```python
from build123d import *

# Parameters (mm, degrees)
SKETCH1_W           = 30
SKETCH1_H           = 20
SKETCH1_H_2         = 2.5
SKETCH1_W_2         = 14
SKETCH1_W_3         = 13.5
SKETCH1_H_3         = 5
SKETCH1_W_4         = 2.5
BOSS_EXTRUDE1_DEPTH = 5
SKETCH1_3_W         = 13.5
SKETCH1_3_H         = 2.5
SKETCH1_3_W_2       = 14
SKETCH1_3_W_3       = 30
SKETCH1_3_W_4       = 2.5
BOSS_EXTRUDE2_DEPTH = 8
SKETCH3_R           = 1.5
CUT_EXTRUDE2_DEPTH  = 2.5
CUT_EXTRUDE3_DEPTH  = 2.5
CUT_EXTRUDE1_DEPTH  = 43.720018727
CUT_EXTRUDE4_DEPTH  = 2.5


with BuildPart() as part:
    # Sketch1 → Boss-Extrude1 (new body)
    with BuildSketch(Plane(origin=(0, 0, 0), x_dir=(1, 0, 0), z_dir=(0, 1, 0))):
        with Locations((-15, -10)):
            Rectangle(SKETCH1_W, SKETCH1_H)
        with Locations((-15, -21.25)):
            Rectangle(SKETCH1_W, SKETCH1_H_2)
        with Locations((-20.5, 1.25)):
            Rectangle(SKETCH1_W_2, SKETCH1_H_2)
        with Locations((-6.75, 1.25)):
            Rectangle(SKETCH1_W_3, SKETCH1_H_2)
        with Locations((-6.75, 5)):
            Rectangle(SKETCH1_W_3, SKETCH1_H_3)
        with Locations((-6.75, 8.75)):
            Rectangle(SKETCH1_W_3, SKETCH1_H_2)
        with Locations((-20.5, 8.75)):
            Rectangle(SKETCH1_W_2, SKETCH1_H_2)
        with Locations((-28.75, 8.75)):
            Rectangle(SKETCH1_W_4, SKETCH1_H_2)
        with Locations((-28.75, 5)):
            Rectangle(SKETCH1_W_4, SKETCH1_H_3)
        with Locations((-28.75, 1.25)):
            Rectangle(SKETCH1_W_4, SKETCH1_H_2)
    boss_extrude1 = extrude(amount=BOSS_EXTRUDE1_DEPTH)

    # Sketch1_3 → Boss-Extrude2 (add)
    with BuildSketch(Plane(origin=(0, 0, 0), x_dir=(1, 0, 0), z_dir=(0, 1, 0))):
        with Locations((-6.75, 1.25)):
            Rectangle(SKETCH1_3_W, SKETCH1_3_H)
        with Locations((-20.5, 1.25)):
            Rectangle(SKETCH1_3_W_2, SKETCH1_3_H)
        with Locations((-15, -21.25)):
            Rectangle(SKETCH1_3_W_3, SKETCH1_3_H)
        with Locations((-28.75, 1.25)):
            Rectangle(SKETCH1_3_W_4, SKETCH1_3_H)
    extrude(amount=BOSS_EXTRUDE2_DEPTH)

    # Sketch3 → Cut-Extrude2 (cut)
    with BuildSketch(Plane(origin=(0, 0, -10), x_dir=(-1, 0, 0), z_dir=(0, 0, -1))):
        with Locations((20.5, 2.5)):
            Circle(SKETCH3_R)
    cut_extrude2 = extrude(amount=-CUT_EXTRUDE2_DEPTH, mode=Mode.SUBTRACT)

    # Sketch4 → Cut-Extrude3 (cut)
    with BuildSketch(Plane(origin=(0, 0, -2.5), x_dir=(-1, 0, 0), z_dir=(0, 0, -1))):
        Polygon((23.675426481, 2.5), (22.08771324, 5.25), (18.91228676, 5.25), (17.324573519, 2.5), (18.91228676, -0.25), (22.08771324, -0.25), align=None)
    cut_extrude3 = extrude(amount=-CUT_EXTRUDE3_DEPTH, mode=Mode.SUBTRACT)

    # Mirror1: Boss-Extrude1, Cut-Extrude2, Cut-Extrude3 across plane
    add(boss_extrude1.mirror(Plane(origin=(0, 0, 10), x_dir=(1, 0, 0), z_dir=(0, 0, -1))))
    add(cut_extrude2.mirror(Plane(origin=(0, 0, 10), x_dir=(1, 0, 0), z_dir=(0, 0, -1))), mode=Mode.SUBTRACT)
    add(cut_extrude3.mirror(Plane(origin=(0, 0, 10), x_dir=(1, 0, 0), z_dir=(0, 0, -1))), mode=Mode.SUBTRACT)

    # Sketch2 → Cut-Extrude1 (cut, through all)
    with BuildSketch(Plane(origin=(0, 5, 0), x_dir=(1, 0, 0), z_dir=(0, 1, 0))):
        with BuildLine():
            ThreePointArc((-13, -10), (-15, -8), (-17, -10))
            Line((-17, -10), (-13, -10))
        make_face()
        with BuildLine():
            Line((-13, -10), (-17, -10))
            ThreePointArc((-17, -10), (-15, -12), (-13, -10))
        make_face()
    extrude(amount=-CUT_EXTRUDE1_DEPTH, mode=Mode.SUBTRACT)

    # Sketch4_3 → Cut-Extrude4 (cut)
    with BuildSketch(Plane(origin=(0, 0, -2.5), x_dir=(-1, 0, 0), z_dir=(0, 0, -1))):
        Polygon((23.675426481, 2.5), (22.08771324, 5.25), (18.91228676, 5.25), (17.324573519, 2.5), (18.91228676, -0.25), (22.08771324, -0.25), align=None)
    extrude(amount=-CUT_EXTRUDE4_DEPTH, mode=Mode.SUBTRACT)


solid = part.part
```
Source: CAD feature listing. Evaluate the final solid. Frame: model axes, mm. A direction names the side the tool comes from. Coordinates: 2 decimals unless noted, no trailing zeros. Loops run counter-clockwise (first coordinate to the right, second up) from the corner with the lowest first, then second, coordinate; pieces in that order, holes last. Notation, with made-up numbers: M -9,-12.75 L -4,-12.75 A18 ccw -4,11.25 Z; hole C 70.25,44.5 d10. An arc over 180 degrees is marked long. Put each result on its own line as item: value. Start each with the question number.
1) Pull-direction query (Y, two-part tool) for faces 1 (the face through (-30, 2, 10)), 2 (the face through (-21, 5.25, -1)), 3 (the face through (-18.13, 3.894, -1.268)); classes: pulls with the +Y half, pulls with the -Y half, needs draft (parallel to the pull), parting line crosses it, or undercut.
2) Cut plane A-A on x = -15. Return the cut outline in (y, z), then the cut area to 3 significant figures.
3) Ray query, L1, parallel to Z at x = -15, y = 2.85; L2, parallel to Y at x = -20.5, z = -8.6; L3, parallel to X at y = 1.5, z = -3. Return the intervals inside material, ascending. Write a range as from..to.
4) Contact query for flat-ended pins moving along their axis: pin 1 Ø1 at (x, z) = (-6, 23.5) entering from +Y; pin 2 Ø1.5 at (x, y) = (-17.5, 6) entering from +Z; pin 3 Ø1.2 at (x, z) = (-21, 21) entering from -Y. Output: stop coordinate, or through.
5) Cut plane C-C on z = 24. Return the cut outline in (x, y), then the cut area to 3 significant figures.
6) Cut plane D-D on x = -20.5. Return the cut outline in (y, z), then the cut area to 3 significant figures.
7) Reachability of faces 4 (the face through (-20, 3, 0)), 5 (the face through (-15, 5, 22.5)), 6 (the face through (-22.2, 2.5, -7.5)) from +Z, -Z, +X, -X, +Y, -Y: full face, straight path, thin tool, end or side. Return the list, or none.
8) Cut plane B-B on y = 7.5. Return the cut outline in (x, z), then the cut area to 3 significant figures.
The answers:
1. face 1: needs draft
1. face 2: pulls with the -Y half
1. face 3: undercut
2. outline: M 0,-10 L 5,-10 L 5,-7.5 L 0,-7.5 Z; M 0,-2.5 L 8,-2.5 L 8,0 L 5,0 L 5,8 L 0,8 Z; M 0,12 L 5,12 L 5,20 L 8,20 L 8,22.5 L 0,22.5 Z; M 0,27.5 L 5,27.5 L 5,30 L 0,30 Z
2. area: 145 mm²
3. L1: z = -10..-7.5, -2.5..8, 12..22.5, 27.5..30
3. L2: y = 0..1, 4..5
3. L3: x = -30..-27.5, -13.5..0
4. pin 1: stops at y = 5
4. pin 2: stops at z = 22.5
4. pin 3: stops at y = 5.25
5. outline: M -30,0 L -27.5,0 L -27.5,5 L -30,5 Z; M -13.5,0 L 0,0 L 0,5 L -13.5,5 Z
5. area: 80.0 mm²
6. outline: M 0,-10 L 1,-10 L 1,-7.5 L 0,-7.5 Z; M 0,0 L 5,0 L 5,20 L 0,20 Z; M 0,27.5 L 1,27.5 L 1,30 L 0,30 Z; M 4,-10 L 5,-10 L 5,-7.5 L 4,-7.5 Z; M 4,27.5 L 5,27.5 L 5,30 L 4,30 Z; M 5.25,-2.5 L 8,-2.5 L 8,0 L 5.25,0 Z; M 5.25,20 L 8,20 L 8,22.5 L 5.25,22.5 Z
6. area: 124 mm²
7. face 4: none
7. face 5: +Y
7. face 6: +Y, -Y
8. outline: M -30,-2.5 L 0,-2.5 L 0,0 L -30,0 Z; M -30,20 L 0,20 L 0,22.5 L -30,22.5 Z
8. area: 150 mm²
